The listing builds one solid part. Answer for the finished solid, in the listing's coordinates (mm). Face numbers are marked on the shaded views. A direction names the side the tool comes from. Give positions to 0.01 mm unless a question says otherwise; leave off trailing zeros. Loops run counter-clockwise (first coordinate to the right, second up) from the corner with the lowest first, then second, coordinate; pieces in that order, holes last. Notation, with made-up numbers: M 44,69.5 L 92,69.5 A23 cw 92,108.5 Z; hole C 69,44.25 d5. An arc over 180 degrees is marked long. One line per item, written item: value. Start each with the question number.
Q1. A cutting plane is placed at D-D, the plane x = -22. Determine the outline of the cut face in (y, z).
Q2. A cutting plane is placed at A-A, the plane z = 0. Determine the outline of the cut face in (x, y) (3 decimals), and give its area (3 significant figures).
Q3. A cutting plane is placed at B-B, the plane y = 11.5. Determine the outline of the cut face in (x, z).
Q4. A cutting plane is placed at C-C, the plane z = 20.5. Determine the outline of the cut face in (x, y) (3 decimals), and give its area (3 significant figures).
Q5. Flat-ended cylindrical pins translate along their axes: pin 1 (5 mm diameter, centred on x = 12.5, z = 24.5, fed in from -Y); pin 2 (8 mm diameter, centred on y = -12.7, z = 12.7, fed in from +X); pin 3 (9.5 mm diameter, centred on x = -12.7, z = -25.4, fed in from +Y). Find the tip coordinate at first contact, or state that the pin passes through.
Q6. Consider L1, parallel to Z at x = -22.4, y = -12.7; L2, parallel to Z at x = 12, y = -23; L3, parallel to Z at x = -23.5, y = 12.7. Determine where each line is inside the solid, lowest interval first.
Q7. For the marked faces 1 and 2, determine the directions among +Z, -Z, +X, -X, +Y, -Y from which every point of the face is accessible in a straight line to the end or side of a thin tool.
from build123d import *

# Parameters (mm, degrees)
BOSS_EXTRUDE1_DEPTH      = 36.5125
BOSS_EXTRUDE1_DEPTH_BACK = 36.5125
CUT_EXTRUDE1_DEPTH       = 65.004725383
CUT_EXTRUDE1_DEPTH_BACK  = 65.004725383
CUT_EXTRUDE2_DEPTH       = 65.004725383
CUT_EXTRUDE2_DEPTH_BACK  = 65.004725383
SKETCH6_R                = 3.5687
SKETCH7_R                = 3.5687
CUT_EXTRUDE3_DEPTH       = 65.004725383


with BuildPart() as part:
    # Sketch4 → Boss-Extrude1 (new, two sides: drawn at the far end of the back side and taken through both)
    with BuildSketch(Plane.XY.offset(-BOSS_EXTRUDE1_DEPTH_BACK)):
        with BuildLine():
            Line((-25.4, 25.4), (-25.4, -25.4))
            Line((-25.4, -25.4), (25.4, -25.4))
            ThreePointArc((25.4, -25.4), (24.001376302, -22.023423698), (20.6248, -20.6248))
            Line((20.6248, -20.6248), (-17.4498, -20.6248))
            ThreePointArc((-17.4498, -20.6248), (-19.69486403, -19.69486403), (-20.6248, -17.4498))
            Line((-20.6248, -17.4498), (-20.6248, 20.6248))
            ThreePointArc((-20.6248, 20.6248), (-22.023423698, 24.001376302), (-25.4, 25.4))
        make_face()
    extrude(amount=BOSS_EXTRUDE1_DEPTH + BOSS_EXTRUDE1_DEPTH_BACK)

    # Sketch5 → Cut-Extrude1 (cut, two sides: drawn at the far end of the back side and taken through both)
    with BuildSketch(Plane(origin=(-20.6248, 0, 0), x_dir=(0, 0, -1), z_dir=(1, 0, 0)).offset(-CUT_EXTRUDE1_DEPTH_BACK)):
        Polygon((-36.5125, -17.4498), (-25.4, 25.4), (-36.5125, 25.4), align=None)
        Polygon((36.5125, 25.4), (25.4, 25.4), (36.5125, -17.4498), align=None)
    extrude(amount=CUT_EXTRUDE1_DEPTH + CUT_EXTRUDE1_DEPTH_BACK, mode=Mode.SUBTRACT)

    # Sketch6 → Cut-Extrude2 (cut, two sides: drawn at the far end of the back side and taken through both)
    with BuildSketch(Plane(origin=(-20.6248, 0, 0), x_dir=(0, 0, -1), z_dir=(1, 0, 0)).offset(-CUT_EXTRUDE2_DEPTH_BACK)):
        with Locations(Location((-12.7, 12.7, 0), (0, 0, 90))):
            Circle(SKETCH6_R)
        with Locations(Location((-12.7, -12.7, 0), (0, 0, 90))):
            Circle(SKETCH6_R)
        with Locations(Location((12.7, -12.7, 0), (0, 0, 90))):
            Circle(SKETCH6_R)
        with Locations(Location((12.7, 12.7, 0), (0, 0, 90))):
            Circle(SKETCH6_R)
    extrude(amount=CUT_EXTRUDE2_DEPTH + CUT_EXTRUDE2_DEPTH_BACK, mode=Mode.SUBTRACT)

    # Sketch7 → Cut-Extrude3 (cut, through all)
    with BuildSketch(Plane(origin=(0, -20.6248, 0), x_dir=(1, 0, 0), z_dir=(0, 1, 0))):
        with Locations(Location((-12.7, 0, 0), (0, 0, 180))):
            Circle(SKETCH7_R)
        with Locations(Location((-12.7, 25.4, 0), (0, 0, 180))):
            Circle(SKETCH7_R)
        with Locations(Location((-12.7, -25.4, 0), (0, 0, 180))):
            Circle(SKETCH7_R)
        with Locations((12.7, -25.4)):
            Circle(SKETCH7_R)
        with Locations((12.7, 25.4)):
            Circle(SKETCH7_R)
        with Locations((12.7, 0)):
            Circle(SKETCH7_R)
    extrude(amount=-CUT_EXTRUDE3_DEPTH, mode=Mode.SUBTRACT)


solid = part.part
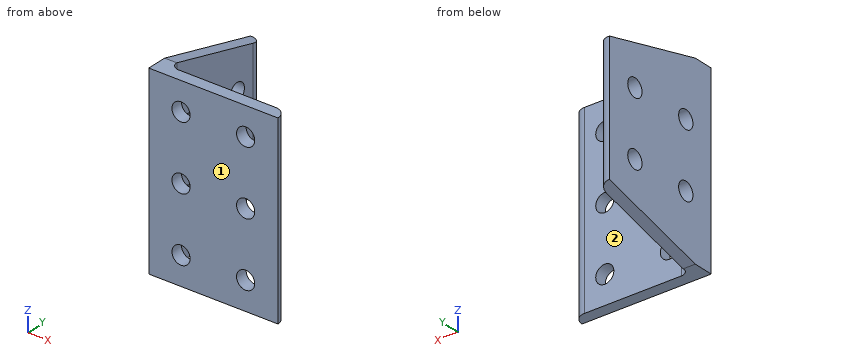
Answer block:
1. outline: M -25.4,-36.51 L -17.45,-36.51 L 23.98,-25.77 L 23.98,25.77 L -17.45,36.51 L -25.4,36.51 Z; hole C -12.7,-12.7 d7.14; hole C -12.7,12.7 d7.14; hole C 12.7,-12.7 d7.14; hole C 12.7,12.7 d7.14
2. outline: M -25.4,-25.4 L -16.269,-25.4 L -16.269,-20.625 L -17.45,-20.625 A3.175 cw -20.625,-17.45 L -20.625,20.625 A4.775 ccw -25.4,25.4 Z; M -9.131,-25.4 L 9.131,-25.4 L 9.131,-20.625 L -9.131,-20.625 Z; M 16.269,-25.4 L 25.4,-25.4 A4.775 ccw 20.625,-20.625 L 16.269,-20.625 Z
2. area: 387 mm^2
3. outline: M -25.4,-29 L -20.62,-29 L -20.62,-16.06 L -25.4,-16.06 Z; M -25.4,-9.34 L -20.62,-9.34 L -20.62,9.34 L -25.4,9.34 Z; M -25.4,16.06 L -20.62,16.06 L -20.62,29 L -25.4,29 Z
4. outline: M -25.4,-25.4 L 25.4,-25.4 A4.775 ccw 20.625,-20.625 L -17.45,-20.625 A3.175 cw -20.625,-17.45 L -20.625,20.625 A4.775 ccw -25.4,25.4 Z
4. area: 455 mm^2
5. pin 1: through
5. pin 2: x = -20.62
5. pin 3: y = -20.62
6. L1: -35.28 to -16.27, -9.13 to 9.13, 16.27 to 35.28
6. L2: -36.51 to -28.9, -21.9 to -3.5, 3.5 to 21.9, 28.9 to 36.51
6. L3: -28.69 to -16.27, -9.13 to 9.13, 16.27 to 28.69
7. face 1: +Z, -Z, +X, -X, -Y
7. face 2: +Z, -Z, +X, +Y
